Job drawing, mm, ordinate dimensions from the low corner. One solid piece. A direction names the side the tool comes from. Give positions to 0.01 mm unless a question says otherwise; leave off trailing zeros. Order: outer loops, then holes, each group sorted by start corner. A loop starts at its lowest first (then second) coordinate and runs counter-clockwise, first axis right, second up. Notation, with made-up numbers: (20, -7.75) - (38, -7.75) arc R19 cw to (38, -3.75) - close; hole circle Ø2 at (71, 53.5). An arc over 180 degrees is marked (long way). One line per item, written item: value.
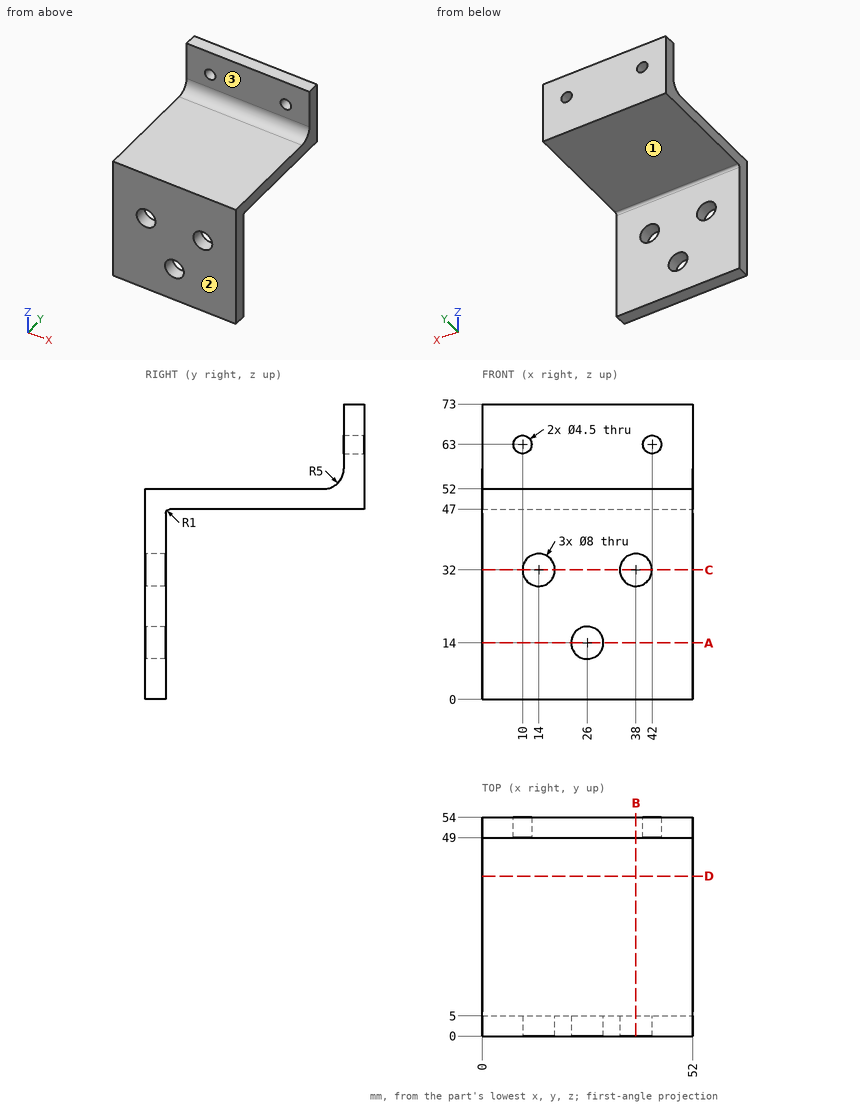
1) Slice it at C-C on z = 32. Write the cut outline in (x, y).
Answer:
outline: (0, 0) - (10, 0) - (10, 5) - (0, 5) - close; (18, 0) - (34, 0) - (34, 5) - (18, 5) - close; (42, 0) - (52, 0) - (52, 5) - (42, 5) - close
2) Which spindle directions (+Z, -Z, +X, -X, +Y, -Y) get a long thin tool onto all of the face, cutting with end or side? Do the marked faces 1, 2 and 3. Say none if no direction does.
Answer:
face 1: -Z, +X, -X, +Y
face 2: +Z, -Z, +X, -X, -Y
face 3: +Z, +X, -X, -Y
3) Drop flat-ended pins along their axis: P1, Ø2, axis at x = 30, z = 37, coming from the +Y side; P2, Ø4, axis at x = 9.5, y = 31, coming from the +Z side; P3, Ø8, axis at x = 28.5, y = 40.5, coming from the -Z side; P4, Ø6, axis at x = 10, z = 63, coming from the +Y side. Give the stop position or say it passes through.
Answer:
P1: stops at y = 5
P2: stops at z = 52
P3: stops at z = 47
P4: stops at y = 54
4) Wall check: line 1 along X through (y, z) = (51.45, 63); line 2 along Z through (x, y) = (14, 2.2); line 3 along Y through (x, z) = (14.5, 8). Give the ranges that are in metal, low to high. Write a range as [from, to].
Answer:
line 1: x = [0, 7.75], [12.25, 39.75], [44.25, 52]
line 2: z = [0, 28], [36, 52]
line 3: y = [0, 5]
5) Slice it at D-D on y = 39.5. Write the cut outline in (x, z).
Answer:
outline: (0, 47) - (52, 47) - (52, 52) - (0, 52) - close
6) Slice it at B-B on x = 38. Write the cut outline in (y, z), then the cut area to 3 significant figures.
Answer:
outline: (0, 0) - (5, 0) - (5, 28) - (0, 28) - close; (0, 36) - (5, 36) - (5, 46) arc R1 cw to (6, 47) - (54, 47) - (54, 73) - (49, 73) - (49, 57) arc R5 cw to (44, 52) - (0, 52) - close
area: 576 mm2
7) Slice it at A-A on z = 14. Write the cut outline in (x, y).
Answer:
outline: (0, 0) - (22, 0) - (22, 5) - (0, 5) - close; (30, 0) - (52, 0) - (52, 5) - (30, 5) - close
